Study the drawing (mm; zero at the part's minimum x, y, z) and answer. A direction names the side the tool comes from. Coordinates: 2 decimals unless noted, no trailing zeros. Order: outer loops, then holes, each group sorted by start corner. A loop starts at its lowest first (then second) coordinate and runs counter-clockwise, first axis right, second up. Notation, with made-up numbers: (47, 31.25) - (62, 31.25) arc R13 ccw to (62, 48.25) - close; hole circle Ø11 at (19.25, 62.5). An arc over 180 degrees is marked (long way). Write item = value, one per line.
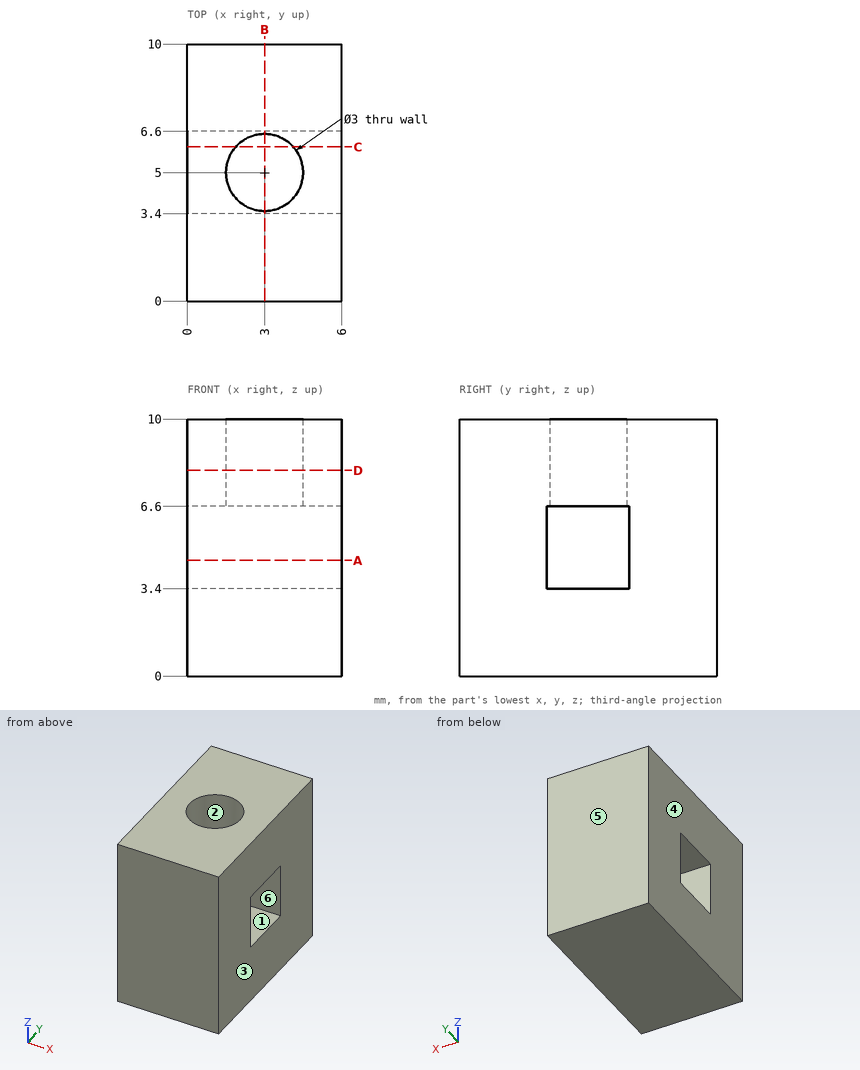
1) For the marked faces 1, 2 and 3, determine the directions among +Z, -Z, +X, -X, +Y, -Y from which every point of the face is accessible in a straight line to the end or side of a thin tool.
Returned:
face_1 = +X, -X
face_2 = +Z
face_3 = +Z, -Z, +X, +Y, -Y
2) A flat-ended cylindrical pin translates along its axis: pin 1 Ø2.5 at (x, y) = (3, 5) entering from +Z. Find the tip coordinate at first contact, or state that the pin passes through.
Returned:
pin_1 = 3.4
3) Determine the mould class of the marked faces 4, 5 and 6 for opening direction Y: pulls with the +Y half, pulls with the -Y half, needs draft (parallel to the pull), parting line crosses it, or undercut.
Returned:
face_4 = needs draft
face_5 = pulls with the +Y half
face_6 = undercut
4) Straight lines are drawn through the part: line 1 along Y through (x, z) = (3, 8.25); line 2 along X through (y, z) = (5, 7.7); line 3 along Z through (x, y) = (4.6, 5). For each, find the intervals that lie inside material, in ascending order. Write a range as from..to.
Returned:
line_1 = 0..3.5, 6.5..10
line_2 = 0..1.5, 4.5..6
line_3 = 0..3.4, 6.6..10
5) The part is cut by section B-B (x = 3). Determine the outline of the cut face in (y, z), and give its area (3 significant figures).
Returned:
outline = (0, 0) - (10, 0) - (10, 10) - (6.5, 10) - (6.5, 6.6) - (6.6, 6.6) - (6.6, 3.4) - (3.4, 3.4) - (3.4, 6.6) - (3.5, 6.6) - (3.5, 10) - (0, 10) - close
area = 79.6 mm^2
6) The part is cut by section D-D (z = 8). Determine the outline of the cut face in (x, y).
Returned:
outline = (0, 0) - (6, 0) - (6, 10) - (0, 10) - close; hole circle Ø3 at (3, 5)
7) The part is cut by section C-C (y = 6). Determine the outline of the cut face in (x, z).
Returned:
outline = (0, 0) - (6, 0) - (6, 3.4) - (0, 3.4) - close; (0, 6.6) - (1.88, 6.6) - (1.88, 10) - (0, 10) - close; (4.12, 6.6) - (6, 6.6) - (6, 10) - (4.12, 10) - close
8) The part is cut by section A-A (z = 4.5). Determine the outline of the cut face in (x, y).
Returned:
outline = (0, 0) - (6, 0) - (6, 3.4) - (0, 3.4) - close; (0, 6.6) - (6, 6.6) - (6, 10) - (0, 10) - close
